Design review of the part built by this model. Coordinates are the model's own, in mm. Face numbers are marked on the shaded views. A direction names the side the tool comes from. Coordinates: 2 decimals unless noted, no trailing zeros. Write each loop counter-clockwise with the first axis right and the second up, starting at its lowest first coordinate (ties: lowest second). Pieces come first, ordered by that corner, then holes. Notation, with made-up numbers: (19, -5.75) -> (50, -5.75) arc R16 cw to (50, 11.25) -> close; hole circle Ø1 at (64, 86.5). An arc over 180 degrees is marked (long way). Answer in a Markdown table with one row per item. Add a question column.
Item 1: Clearance check with flat-ended pins moving along their axes: P1, Ø1, axis at y = -7, z = 123, coming from the -X side; P2, Ø1.5, axis at x = -101, z = 124.5, coming from the -Y side; P3, Ø5, axis at x = -176, y = -15.5, coming from the -Z side. State where each tip first meets the part, or that it passes through.
Item 2: To check wall thickness, follow line 1 (Y direction, x = -176, z = 123.25); line 2 (Y direction, x = -122, z = 118.75); line 3 (Z direction, x = -183, y = -12.25). State the ranges of each line that lie inside material, in increasing order.
Item 3: Take a section at C-C, the plane x = -198. Write out the cut boundary in (y, z).
Item 4: Take a section at A-A, the plane y = -18. Write out the cut boundary in (x, z).
Item 5: Take a section at D-D, the plane z = 129.5. Write out the cut boundary in (x, y).
Item 6: Take a section at B-B, the plane z = 124. Write out the cut boundary in (x, y), and give its area (3 significant figures).
Item 7: For the marked faces 1, 2, 3 and 4, list the 3-axis set-ups (+Z, -Z, +X, -X, +Y, -Y) from which the entire face can be reached by the end or side of a thin tool; tool diameter is ignored.
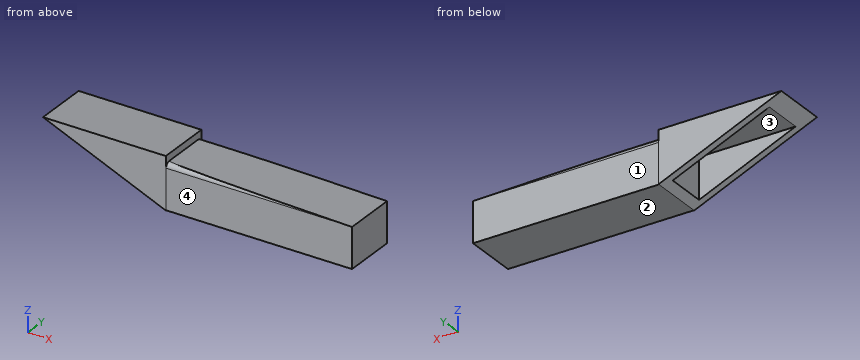
from build123d import *

# Parameters (mm, degrees)
BOSS_EXTRU_1_DEPTH              = 23
ENL_V_MAT_EXTRU_2_DEPTH         = 47.939769219
ENL_V_DE_MAT_EXTRU_MINCE1_DEPTH = 78.627208506


with BuildPart() as part:
    # Esquisse3 → Boss.-Extru.1 (new body)
    with BuildSketch(Plane(origin=(0, 0, 0), x_dir=(1, 0, 0), z_dir=(0, 1, 0))):
        Polygon((-209.233275871, -136.906813661), (-157.293506651, -114.887808395), (-78.666298145, -114.887808395), (-78.666298145, -131.906813661), (-157.293506651, -133.906813661), (-157.293506651, -136.906813661), align=None)
    extrude(amount=-BOSS_EXTRU_1_DEPTH)

    # Esquisse5 → Enlèv. mat.-Extru.2 (cut)
    with BuildSketch(Plane.YZ.offset(-209.233275871)):
        Polygon((-20, 133.906813661), (-20, 117.887808395), (-20, 114.887808395), (-3, 114.887808395), (-3, 117.887808395), (-3, 133.906813661), align=None)
    extrude(amount=ENL_V_MAT_EXTRU_2_DEPTH, mode=Mode.SUBTRACT)

    # Esquisse6 → Enlèv. de mat.-Extru.-Mince1 (cut)
    with BuildSketch(Plane(origin=(-78.666298145, 0, 0), x_dir=(0, 0, -1), z_dir=(1, 0, 0))):
        with BuildLine():
            Line((-134.906813661, -20.8), (-134.906813661, -1.954954154))
            ThreePointArc((-134.906813661, -1.954954154), (-133.945165816, 0.010427616), (-131.904561119, 0.8))
            Line((-131.904561119, 0.8), (-113.24643884, 0.8))
            Line((-113.24643884, 0.8), (-113.24643884, -23.8))
            Line((-113.24643884, -23.8), (-131.906813661, -23.8))
            ThreePointArc((-131.906813661, -23.8), (-134.028134004, -22.921320344), (-134.906813661, -20.8))
        make_face()
        with BuildLine():
            Line((-133.906813661, -20.8), (-133.906813661, -2))
            ThreePointArc((-133.906813661, -2), (-133.254765726, -0.713386594), (-131.906813661, -0.2))
            Line((-131.906813661, -0.2), (-114.24643884, -0.2))
            Line((-114.24643884, -0.2), (-114.24643884, -22.8))
            Line((-114.24643884, -22.8), (-131.906813661, -22.8))
            ThreePointArc((-131.906813661, -22.8), (-133.321027223, -22.214213562), (-133.906813661, -20.8))
        make_face(mode=Mode.SUBTRACT)
    extrude(amount=-ENL_V_DE_MAT_EXTRU_MINCE1_DEPTH, mode=Mode.SUBTRACT)


solid = part.part
Answers:
| question | item | result |
|---|---|---|
| 1 | P1 | stops at x = -161.29 |
| 1 | P2 | stops at y = -22.8 |
| 1 | P3 | stops at z = 133.91 |
| 2 | line 1 | y = -23 to -20, -3 to 0 |
| 2 | line 2 | y = -22.8 to -0.2 |
| 2 | line 3 | z = 133.91 to 136.91 |
| 3 | outline | (-23, 132.14) -> (-20, 132.14) -> (-20, 133.91) -> (-3, 133.91) -> (-3, 132.14) -> (0, 132.14) -> (0, 136.91) -> (-23, 136.91) -> close |
| 4 | outline | (-209.23, 136.91) -> (-202.16, 133.91) -> (-161.29, 133.91) -> (-161.29, 116.58) -> (-157.29, 114.89) -> (-78.67, 114.89) -> (-78.67, 131.91) -> (-157.29, 133.91) -> (-157.29, 136.91) -> close |
| 5 | outline | (-191.76, -23) -> (-157.29, -23) -> (-157.29, -22.8) -> (-78.67, -22.8) -> (-78.67, -0.2) -> (-157.29, -0.2) -> (-157.29, 0) -> (-191.76, 0) -> (-191.76, -3) -> (-161.29, -3) -> (-161.29, -20) -> (-191.76, -20) -> close |
| 6 | outline | (-178.79, -23) -> (-157.29, -23) -> (-157.29, -22.8) -> (-78.67, -22.8) -> (-78.67, -0.2) -> (-157.29, -0.2) -> (-157.29, 0) -> (-178.79, 0) -> (-178.79, -3) -> (-161.29, -3) -> (-161.29, -20) -> (-178.79, -20) -> close |
| 6 | area | 1,970 mm^2 |
| 7 | face 1 | +Z, -Z, +X, +Y |
| 7 | face 2 | -Z, +X, -X, +Y, -Y |
| 7 | face 3 | -Z, -X |
| 7 | face 4 | +Z, -Z, +X, -Y |
